from build123d import *

# Parameters (mm, degrees)
EXTRUDE_1_DEPTH      = 8
CUT_EXTRUDE_1_DEPTH  = 8.6
EXTRUDE_2_DEPTH      = 8
EXTRUDE_3_DEPTH      = 10
SKETCH_7_R           = 5.75
CUT_EXTRUDE_2_DEPTH  = 22
EXTRUDE_5_DEPTH      = 26
CUT_EXTRUDE_4_DEPTH  = 21
CHAMFER_6_SIZE       = 5
CHAMFER_8_SIZE       = 10
SKETCH_13_W          = 210
SKETCH_13_H          = 10
CUT_EXTRUDE_5_DEPTH  = 15
SKETCH_14_W          = 160
SKETCH_14_H          = 5
CUT_EXTRUDE_6_DEPTH  = 10
SKETCH_16_R          = 2
CUT_EXTRUDE_7_DEPTH  = 10
SKETCH_18_W          = 109.386418102
SKETCH_18_H          = 16
EXTRUDE_7_DEPTH      = 2
CHAMFER_10_SIZE      = 2
SKETCH_32_W          = 100
SKETCH_32_H          = 25
CUT_EXTRUDE_16_DEPTH = 3
SKETCH_33_W          = 3
SKETCH_33_H          = 25
CUT_EXTRUDE_17_DEPTH = 1003
SKETCH_34_W          = 1.5
SKETCH_34_H          = 25
CUT_EXTRUDE_19_DEPTH = 3
SKETCH_36_W          = 111.215468024
SKETCH_36_H          = 1.5
CUT_EXTRUDE_20_DEPTH = 3
CUT_EXTRUDE_21_DEPTH = 3
SKETCH_38_W          = 1.5
SKETCH_38_H          = 31
CUT_EXTRUDE_22_DEPTH = 1003


with BuildPart() as part:
    # 草图1 → 凸台-拉伸1 (new body)
    with BuildSketch(Plane.XY):
        Polygon((-60, 0), (60, 0), (115, 270), (-115, 270), align=None)
    extrude(amount=EXTRUDE_1_DEPTH)

    # 草图2 → 切除-拉伸1 (cut)
    with BuildSketch(Plane.XY.offset(8)):
        with BuildLine():
            Line((0.005000474, 0.310000947), (0, 0.3))
            Line((0, 0.3), (17.48870838, 0.3))
            Line((17.48870838, 0.3), (12.108893566, 26.71))
            Line((12.108893566, 26.71), (0, 26.71))
            ThreePointArc((0, 26.71), (-13.199999763, 13.507499763), (0.005000474, 0.310000947))
        make_face()
    extrude(amount=-CUT_EXTRUDE_1_DEPTH, mode=Mode.SUBTRACT)

    # 草图5 → 凸台-拉伸2 (add)
    with BuildSketch(Plane(origin=(0, 0, 0), x_dir=(-1, 0, 0), z_dir=(0, 0, -1))):
        Polygon((60, 0), (115, 270), (-115, 270), (-60, 0), align=None)
    extrude(amount=EXTRUDE_2_DEPTH)

    # 草图6 → 凸台-拉伸3 (add)
    with BuildSketch(Plane.XY.offset(8)):
        Polygon((-115, 270), (-60, 0), (60, 0), (115, 270), align=None)
    extrude(amount=EXTRUDE_3_DEPTH)

    # 草图7 → 切除-拉伸2 (cut)
    with BuildSketch(Plane.XY.offset(18)):
        with Locations((0, 13.51)):
            Circle(SKETCH_7_R)
    extrude(amount=-CUT_EXTRUDE_2_DEPTH, mode=Mode.SUBTRACT)

    # 草图9 → 凸台-拉伸5 (add)
    with BuildSketch(Plane.XY.offset(18)):
        Polygon((-57.962962963, -10), (-60, 0), (60, 0), (57.962962963, -10), align=None)
    extrude(amount=-EXTRUDE_5_DEPTH)

    # 草图12 → 切除-拉伸4 (cut)
    with BuildSketch(Plane.XY.offset(-8)):
        Polygon((54.693209051, 0), (-54.693209051, 0), (-52.656172014, -10), (52.656172014, -10), align=None)
    extrude(amount=CUT_EXTRUDE_4_DEPTH, mode=Mode.SUBTRACT)

    # 倒角6
    chamfer_6_edges = [part.edges().sort_by_distance(p)[0] for p in [
        (0, 0, -8),
    ]]
    chamfer(chamfer_6_edges, length=CHAMFER_6_SIZE)

    # 倒角8
    chamfer_8_edges = [part.edges().sort_by_distance(p)[0] for p in [
        (55.309567488, -10, -8),
        (-55.309567488, -10, -8),
    ]]
    chamfer(chamfer_8_edges, length=CHAMFER_8_SIZE)

    # 草图13 → 切除-拉伸5 (cut)
    with BuildSketch(Plane(origin=(0, 270, 0), x_dir=(1, 0, 0), z_dir=(0, 1, 0))):
        with Locations((0, -5)):
            Rectangle(SKETCH_13_W, SKETCH_13_H)
    extrude(amount=-CUT_EXTRUDE_5_DEPTH, mode=Mode.SUBTRACT)

    # 草图14 → 切除-拉伸6 (cut)
    with BuildSketch(Plane.XY.offset(18)):
        with Locations((0, 173.51)):
            Rectangle(SKETCH_14_W, SKETCH_14_H)
    extrude(amount=-CUT_EXTRUDE_6_DEPTH, mode=Mode.SUBTRACT)

    # 草图16 → 切除-拉伸7 (cut)
    with BuildSketch(Plane.XY.offset(18)):
        with BuildLine():
            ThreePointArc((-88.677124344, 235), (-90, 238.5), (-91.322875656, 235))
            Line((-91.322875656, 235), (-88.677124344, 235))
        make_face()
        with BuildLine():
            ThreePointArc((91.322875656, 235), (90, 238.5), (88.677124344, 235))
            Line((88.677124344, 235), (91.322875656, 235))
        make_face()
        with BuildLine():
            ThreePointArc((65.822875656, 235), (64.5, 238.5), (63.177124344, 235))
            Line((63.177124344, 235), (65.822875656, 235))
        make_face()
        with BuildLine():
            ThreePointArc((-63.177124344, 235), (-64.5, 238.5), (-65.822875656, 235))
            Line((-65.822875656, 235), (-63.177124344, 235))
        make_face()
        with Locations((-77.25, 255.6425573)):
            Circle(SKETCH_16_R)
        with Locations((77.25, 255.6425573)):
            Circle(SKETCH_16_R)
        with Locations((-55, 154.1525573)):
            Circle(SKETCH_16_R)
        with Locations((-67.75, 135.01)):
            Circle(SKETCH_16_R)
        with Locations((-42.25, 135.01)):
            Circle(SKETCH_16_R)
        with Locations((42.25, 135.01)):
            Circle(SKETCH_16_R)
        with Locations((67.75, 135.01)):
            Circle(SKETCH_16_R)
        with Locations((55, 154.1525573)):
            Circle(SKETCH_16_R)
    extrude(amount=-CUT_EXTRUDE_7_DEPTH, mode=Mode.SUBTRACT)

    # 草图18 → 凸台-拉伸7 (add)
    with BuildSketch(Plane.XZ):
        with Locations((0, 5)):
            Rectangle(SKETCH_18_W, SKETCH_18_H)
    extrude(amount=EXTRUDE_7_DEPTH)

    # 倒角10
    chamfer_10_edges = [part.edges().sort_by_distance(p)[0] for p in [
        (0, -2, -3),
    ]]
    chamfer(chamfer_10_edges, length=CHAMFER_10_SIZE - 0.0001)  # a hair under: the kernel refuses the full size

    # 草图32 → 切除-拉伸16 (cut)
    with BuildSketch(Plane(origin=(0, 0, -8), x_dir=(-1, 0, 0), z_dir=(0, 0, -1))):
        with Locations((-46.363148148, 206.34047939)):
            Rectangle(SKETCH_32_W, SKETCH_32_H)
    extrude(amount=-CUT_EXTRUDE_16_DEPTH, mode=Mode.SUBTRACT)

    # 草图33 → 切除-拉伸17 (cut)
    with BuildSketch(Plane(origin=(-3.636851852, 0, 0), x_dir=(0, 0, -1), z_dir=(1, 0, 0))):
        with Locations((6.5, 206.34047939)):
            Rectangle(SKETCH_33_W, SKETCH_33_H)
    extrude(amount=CUT_EXTRUDE_17_DEPTH, mode=Mode.SUBTRACT)

    # 草图34 → 切除-拉伸19 (cut)
    with BuildSketch(Plane(origin=(-3.636851852, 0, 0), x_dir=(0, 0, -1), z_dir=(1, 0, 0))):
        with Locations((5.75, 206.34047939)):
            Rectangle(SKETCH_34_W, SKETCH_34_H)
    extrude(amount=-CUT_EXTRUDE_19_DEPTH, mode=Mode.SUBTRACT)

    # 草图36 → 切除-拉伸20 (cut)
    with BuildSketch(Plane.XZ.offset(-218.84047939)):
        with Locations((48.97088216, -5.75)):
            Rectangle(SKETCH_36_W, SKETCH_36_H)
    extrude(amount=-CUT_EXTRUDE_20_DEPTH, mode=Mode.SUBTRACT)

    # 草图37 → 切除-拉伸21 (cut)
    with BuildSketch(Plane(origin=(0, 193.84047939, 0), x_dir=(1, 0, 0), z_dir=(0, 1, 0))):
        Polygon((-6.636851852, 6.5), (-6.636851852, 5), (99.486023579, 5), (99.486023579, 6.5), (-3.636851852, 6.5), align=None)
    extrude(amount=-CUT_EXTRUDE_21_DEPTH, mode=Mode.SUBTRACT)

    # 草图38 → 切除-拉伸22 (cut)
    with BuildSketch(Plane(origin=(-6.636851852, 0, 0), x_dir=(0, 0, -1), z_dir=(1, 0, 0))):
        with Locations((5.75, 206.34047939)):
            Rectangle(SKETCH_38_W, SKETCH_38_H)
    extrude(amount=CUT_EXTRUDE_22_DEPTH, mode=Mode.SUBTRACT)


solid = part.part
Work out the finished part from the listing and answer in its coordinate system (mm). A direction names the side the tool comes from. Give positions to 0.01 mm unless a question says otherwise; leave off trailing zeros. Order: outer loops, then holes, each group sorted by start corner. A loop starts at its lowest first (then second) coordinate and runs counter-clockwise, first axis right, second up. Notation, with made-up numbers: (36.5, -2) -> (86.5, -2) arc R37 cw to (86.5, 37) -> close; hole circle Ø8 at (69.5, -9.5). An arc over 180 degrees is marked (long way). Answer as a JSON object with one key per item and string values. Group by question number.
1. The mould has two halves that part along X. Classify faces 1 (the flat face through (48, 207, -5)), 2 (the cylindrical face through (-13.197, 13.798, 4.056)), 3 (the flat face through (9, 0.3, 4)): released by +X, released by -X, zero draft, split by the parting line, or undercut.
2. Consider line 1 along Y through (x, z) = (-55, 12); line 2 along Y through (x, z) = (0, 13.75); line 3 along Y through (x, z) = (32.5, 13.5). Determine where each line is inside the solid, lowest interval first. Write a range as [from, to].
3. Section B-B on y = 13.51 is taken. Determine the outline of the cut face in (x, z).
4. Section D-D on y = 246 is taken. Determine the outline of the cut face in (x, z).
5. Section C-C on x = -99 is taken. Determine the outline of the cut face in (y, z).
6. A tool of negligible diameter and unlimited length cuts with its end or side. For faces 4 (the flat face through (6, 26.71, 4)), 5 (the flat face through (0, 14, -4)), 6 (the flat face through (41, 191, -6.5)), 7 (the flat face through (-1, 263, 10)), from which of +Z, -Z, +X, -X, +Y, -Y can it reach the whole face along a straight path? Write none if from no direction.
7. Flat-ended cylindrical pins translate along their axes: pin 1 Ø3 at (y, z) = (261, 5.5) entering from -X; pin 2 Ø3 at (y, z) = (23.5, 12.5) entering from -X; pin 3 Ø8 at (y, z) = (113.5, 4) entering from -X. Find the tip coordinate at first contact, or state that the pin passes through.
Result sheet:
{
 "1": {"face 1": "zero draft", "face 2": "undercut", "face 3": "undercut"},
 "2": {"line 1": "y = [-10, 152.15], [156.15, 171.01], [176.01, 270]", "line 2": "y = [-10, 7.76], [19.26, 171.01], [176.01, 270]", "line 3": "y = [-10, 171.01], [176.01, 270]"},
 "3": {"outline": "(-62.75, -8) -> (62.75, -8) -> (62.75, 18) -> (5.75, 18) -> (5.75, 8) -> (14.8, 8) -> (14.8, 0) -> (5.75, 0) -> (5.75, -4) -> (-5.75, -4) -> (-5.75, 0) -> (-13.2, 0) -> (-13.2, 8) -> (-5.75, 8) -> (-5.75, 18) -> (-62.75, 18) -> close"},
 "4": {"outline": "(-110.11, -8) -> (110.11, -8) -> (110.11, 18) -> (-110.11, 18) -> close"},
 "5": {"outline": "(191.45, -8) -> (270, -8) -> (270, 0) -> (255, 0) -> (255, 10) -> (270, 10) -> (270, 18) -> (191.45, 18) -> close"},
 "6": {"face 4": "none", "face 5": "+Z", "face 6": "+X", "face 7": "+Y"},
 "7": {"pin 1": "stops at x = -113.47", "pin 2": "stops at x = -65.09", "pin 3": "stops at x = -83.94"}
}
